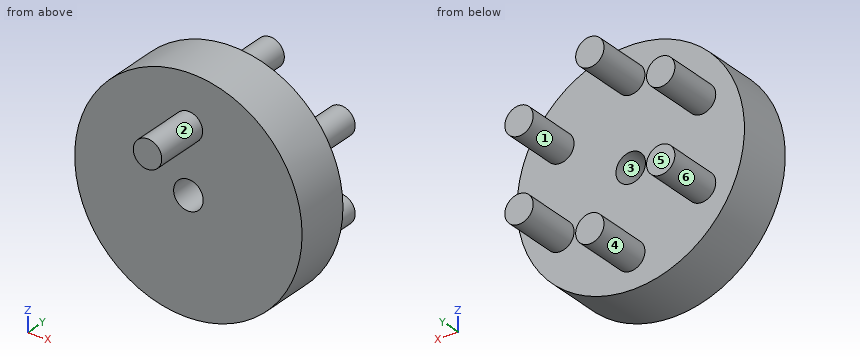
```python
from build123d import *

# Parameters (mm, degrees)
F0_R     = 25.4
F1_DEPTH = 12.7
F2_R     = 3.302
F3_DEPTH = 12.7
F4_R     = 3.175
F5_DEPTH = 12.7
F6_R     = 3.169132
F7_DEPTH = 12.7


with BuildPart() as f1:
    # F0 (on Front) → F1 (new body)
    with BuildSketch(Plane.XZ):
        Circle(F0_R)
    extrude(amount=F1_DEPTH)

    # F2 (on face) → F3 (cut)
    with BuildSketch(Plane.XZ.offset(12.7)):
        Circle(F2_R)
    extrude(amount=-F3_DEPTH, mode=Mode.SUBTRACT)

    # F4 (on face) → F5 (join)
    with BuildSketch(Plane.XZ.offset(12.7)):
        with Locations((0, 14.211592)):
            Circle(F4_R)
    extrude(amount=F5_DEPTH)

    # F6 (on face) → F7 (join)
    with BuildSketch(Plane(origin=(0, 0, 0), x_dir=(-1, 0, 0), z_dir=(0, 1, 0))):
        with Locations((0, 18.275665)):
            Circle(F6_R)
        with Locations((-15.82719, 9.137833)):
            Circle(F6_R)
        with Locations((-15.82719, -9.137833)):
            Circle(F6_R)
        with Locations((0, -18.275665)):
            Circle(F6_R)
        with Locations((15.82719, -9.137833)):
            Circle(F6_R)
        with Locations((15.82719, 9.137833)):
            Circle(F6_R)
    extrude(amount=F7_DEPTH)


solid = f1.part
```
Input: part model. Units: mm. Frame: model coordinates. Face numbers are marked on the shaded views. A direction names the side the tool comes from. Coordinates: 2 decimals unless noted, no trailing zeros. Loops run counter-clockwise (first coordinate to the right, second up) from the corner with the lowest first, then second, coordinate; pieces in that order, holes last. Notation, with made-up numbers: (16, 51.25) -> (49, 51.25) arc R29 ccw to (49, 85.25) -> close; hole circle Ø5 at (-38, 58). An arc over 180 degrees is marked (long way). Use a Markdown table: item, result.
1) Access query for the marked faces 1, 2 and 3. Directions: +Z, -Z, +X, -X, +Y, -Y. A direction counts if a zero-diameter tool reaches every point of the face in a straight line with its end or side. Return the directions, or none.
Results found:
| item | result |
|---|---|
| face 1 | +Y |
| face 2 | -Y |
| face 3 | +Y, -Y |
2) Pull-direction query (X, two-part tool) for the marked faces 4, 5 and 6; classes: released by +X, released by -X, zero draft, split by the parting line, or undercut.
Results found:
| item | result |
|---|---|
| face 4 | split by the parting line |
| face 5 | zero draft |
| face 6 | undercut |
3) Contact query for flat-ended pins moving along their axis: pin 1 (4 mm diameter, centred on x = -6.5, y = -9, fed in from +Z); pin 2 (4 mm diameter, centred on y = 7.5, z = 12, fed in from -X); pin 3 (5 mm diameter, centred on y = 1.5, z = 5.5, fed in from -X); pin 4 (4 mm diameter, centred on x = 0, z = 0, fed in from -Y). Output: stop coordinate, or through.
Results found:
| item | result |
|---|---|
| pin 1 | stops at z = 25 |
| pin 2 | stops at x = -18.88 |
| pin 3 | stops at x = -25.16 |
| pin 4 | passes through |
4) Cut plane B-B (z = 0). Return the cut outline in (x, y), then the cut area to 3 significant figures.
Results found:
| item | result |
|---|---|
| outline | (-25.4, -12.7) -> (-3.3, -12.7) -> (-3.3, 0) -> (-25.4, 0) -> close; (3.3, -12.7) -> (25.4, -12.7) -> (25.4, 0) -> (3.3, 0) -> close |
| area | 561 mm2 |
5) Cut plane C-C (y = 3). Return the cut outline in (x, z).
Results found:
| item | result |
|---|---|
| outline | circle Ø6.34 at (-15.83, -9.14); circle Ø6.34 at (-15.83, 9.14); circle Ø6.34 at (0, -18.28); circle Ø6.34 at (0, 18.28); circle Ø6.34 at (15.83, -9.14); circle Ø6.34 at (15.83, 9.14) |
6) Material intervals for line 1 along Z through (x, y) = (0, -5); line 2 along Z through (x, y) = (0, 4); line 3 along Y through (x, z) = (-4.5, 1.5), sorted ascending. Write a range as from..to.
Results found:
| item | result |
|---|---|
| line 1 | z = -25.4..-3.3, 3.3..25.4 |
| line 2 | z = -21.44..-15.11, 15.11..21.44 |
| line 3 | y = -12.7..0 |
7) Cut plane A-A (x = 0). Return the cut outline in (y, z), then the cut area to 3 significant figures.
Results found:
| item | result |
|---|---|
| outline | (-25.4, 11.04) -> (-12.7, 11.04) -> (-12.7, 3.3) -> (0, 3.3) -> (0, 15.11) -> (12.7, 15.11) -> (12.7, 21.44) -> (0, 21.44) -> (0, 25.4) -> (-12.7, 25.4) -> (-12.7, 17.39) -> (-25.4, 17.39) -> close; (-12.7, -25.4) -> (0, -25.4) -> (0, -21.44) -> (12.7, -21.44) -> (12.7, -15.11) -> (0, -15.11) -> (0, -3.3) -> (-12.7, -3.3) -> close |
| area | 803 mm2 |
8) Cut plane D-D (y = -4). Return the cut outline in (x, z), then the cut area to 3 significant figures.
Results found:
| item | result |
|---|---|
| outline | circle Ø50.8 at (0, 0); hole circle Ø6.6 at (0, 0) |
| area | 1,990 mm2 |
